```python
from build123d import *

# Parameters (mm, degrees)
ESBO_O1_R                = 3.175
RESSALTO_EXTRUS_O1_DEPTH = 11.1125
ESBO_O2_R                = 4.9609375
CORTE_EXTRUS_O1_DEPTH    = 7.9375
FILETE1_R                = 0.5


with BuildPart() as part:
    # Esboço1 → Ressalto-extrusão1 (new body)
    with BuildSketch(Plane.XY):
        Polygon((3.553451716, 6.197269154), (-3.590266663, 6.176014034), (-7.143718379, -0.021255119), (-3.553451716, -6.197269154), (3.590266663, -6.176014034), (7.143718379, 0.021255119), align=None)
        Circle(ESBO_O1_R, mode=Mode.SUBTRACT)
    extrude(amount=RESSALTO_EXTRUS_O1_DEPTH)

    # Esboço2 → Corte-extrusão1 (cut)
    with BuildSketch(Plane(origin=(0, 0, 0), x_dir=(-1, 0, 0), z_dir=(0, 0, -1))):
        Circle(ESBO_O2_R)
    extrude(amount=-CORTE_EXTRUS_O1_DEPTH, mode=Mode.SUBTRACT)

    # Filete1
    filete1_edges = [part.edges().sort_by_distance(p)[0] for p in [
        (-3.175, 0, 11.1125),
    ]]
    fillet(filete1_edges, radius=FILETE1_R)

    # Esboço4 → Corte-Revolução4 (revolve, cut)
    with BuildSketch(Plane(origin=(0, 0, 0), x_dir=(1, 0, 0), z_dir=(0, 1, 0)), mode=Mode.PRIVATE) as corte_revolu_o4_sk:
        Polygon((6.409669222, -16.266104521), (6.409669222, -11.2125), (9.269615278, -8.352553944), (9.269615278, -16.266104521), align=None)
        Polygon((6.409669222, 5.153604521), (9.269615278, 5.153604521), (9.269615278, -2.759946056), (6.409669222, 0.1), align=None)
    revolve(corte_revolu_o4_sk.sketch.rotate(Axis((0, 0, 23.395635865), (0, 0, -1)), 180), axis=Axis((0, 0, 23.395635865), (0, 0, -1)), mode=Mode.SUBTRACT)


solid = part.part
```
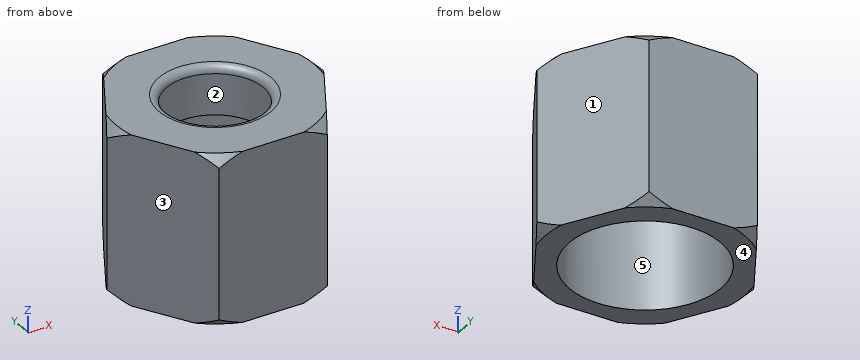
Here's how the part is built. I have some questions about the finished solid (model axes, mm). Face numbers are marked on the shaded views. A direction names the side the tool comes from. Give positions to 0.01 mm unless a question says otherwise; leave off trailing zeros. Order: outer loops, then holes, each group sorted by start corner. A loop starts at its lowest first (then second) coordinate and runs counter-clockwise, first axis right, second up. Notation, with made-up numbers: M 22,-36 L 44,-36 A23 ccw 44,-2 Z; hole C 80,32.25 d5. An arc over 180 degrees is marked long. Use a Markdown table: item, result. Add a question column.
1. I need wall thicknesses on probe 1 along Y at (x, z) = (2.25, 1.5); probe 2 along Z at (x, y) = (4, 0); probe 3 along Y at (x, z) = (0, 2.5). Which ranges of each line are inside material? Lowest first, please. Write a range as from..to.
2. Suppose I cut it at A-A (z = 9.75). List the corners of the cut face in (x, y) for me (3 decimals), and give its area (3 significant figures).
3. On a 3-axis mill with a long thin cutter (end or side, diameter ignored), from which of +Z, -Z, +X, -X, +Y, -Y can I reach the whole of each face in a straight line? I mean the marked faces 4 and 5. Say none if no direction works.
4. Suppose I cut it at C-C (y = -4). List the corners of the cut face in (x, z) for me, and give its area (3 significant figures).
5. Suppose I cut it at D-D (z = 4). List the corners of the cut face in (x, y) for me, and give its area (3 significant figures).
6. For pin 1 Ø3 at (x, y) = (-1.5, -1.5) entering from -Z; pin 2 Ø3 at (x, z) = (-5.5, 5.5) entering from -Y; pin 3 Ø2 at (y, z) = (-3.5, 2) entering from -X, each with a flat end and sliding along its axis, tell me the tip position at first contact or that it passes through.
7. Suppose I cut it at B-B (x = 0). List the corners of the cut face in (y, z) for me (1 decimal).
8. If we mould it in two halves opening along X, with no side actions, what happens to the marked faces 1, 2 and 3? For each: +X half, -X half, draft (parallel to the pull), parting line (faces both ways), or undercut.
Results list:
| question | item | result |
|---|---|---|
| 1 | probe 1 | y = -6.18..-4.42, 4.42..6.19 |
| 1 | probe 2 | z = 7.94..11.11 |
| 1 | probe 3 | y = -6.19..-4.96, 4.96..6.19 |
| 2 | outline | M -7.144,-0.021 L -3.553,-6.197 L 3.59,-6.176 L 7.144,0.021 L 3.553,6.197 L -3.59,6.176 Z; hole C 0,0 d6.35 |
| 2 | area | 101 mm² |
| 3 | face 4 | -Z, +X, -X, +Y, -Y |
| 3 | face 5 | -Z |
| 4 | outline | M -4.83,0 L -2.93,0 L -2.93,7.94 L 2.93,7.94 L 2.93,0 L 4.84,0 L 4.84,11.11 L -4.83,11.11 Z |
| 4 | area | 60.9 mm² |
| 5 | outline | M -7.14,-0.02 L -3.55,-6.2 L 3.59,-6.18 L 7.14,0.02 L 3.55,6.2 L -3.59,6.18 Z; hole C 0,0 d9.92 |
| 5 | area | 55.3 mm² |
| 6 | pin 1 | stops at z = 7.94 |
| 6 | pin 2 | stops at y = -5.43 |
| 6 | pin 3 | stops at x = -5.7 |
| 7 | outline | M -6.2,0 L -5,0 L -5,7.9 L -3.2,7.9 L -3.2,10.6 A0.5 ccw -3.7,11.1 L -6.2,11.1 Z; M 3.2,7.9 L 5,7.9 L 5,0 L 6.2,0 L 6.2,11.1 L 3.7,11.1 A0.5 ccw 3.2,10.6 Z |
| 8 | face 1 | +X half |
| 8 | face 2 | undercut |
| 8 | face 3 | -X half |
